Input: dimensioned drawing with shaded views. Units: mm. Origin: part minimum x, y, z. A direction names the side the tool comes from. Round coordinates to 2 decimals unless told otherwise and drop trailing zeros. Order: outer loops, then holes, each group sorted by start corner. A loop starts at its lowest first (then second) coordinate and runs counter-clockwise, first axis right, second up. Notation, with made-up numbers: M -6.75,-16.75 L 51.25,-16.75 A38 ccw 51.25,21.25 Z; hole C 89,27.25 d10. An arc over 180 degrees is marked long. Use one line per item in the form item = value. Start each with the question number.
Q1. Section D-D (z = 15). Return the cut outline in (x, y).
Q2. Reachability of the marked faces 1 and 2 from +Z, -Z, +X, -X, +Y, -Y: full face, straight path, thin tool, end or side. Return the list, or none.
Q3. Material intervals for probe 1 along Y at (x, z) = (29, 3.25); probe 2 along Z at (x, y) = (13, 50); probe 3 along X at (y, z) = (34, 16), sorted ascending.
Q4. Section C-C (z = 44). Return the cut outline in (x, y).
Q5. Section A-A (x = 29). Return the cut outline in (y, z).
Q6. Contact query for flat-ended pins moving along their axis: pin 1 (10 mm diameter, centred on x = 12.5, z = 22.5, fed in from +Y); pin 2 (1 mm diameter, centred on x = 50.5, y = 19, fed in from +Z); pin 3 (1 mm diameter, centred on y = 50, z = 25.5, fed in from -X). Output: stop coordinate, or through.
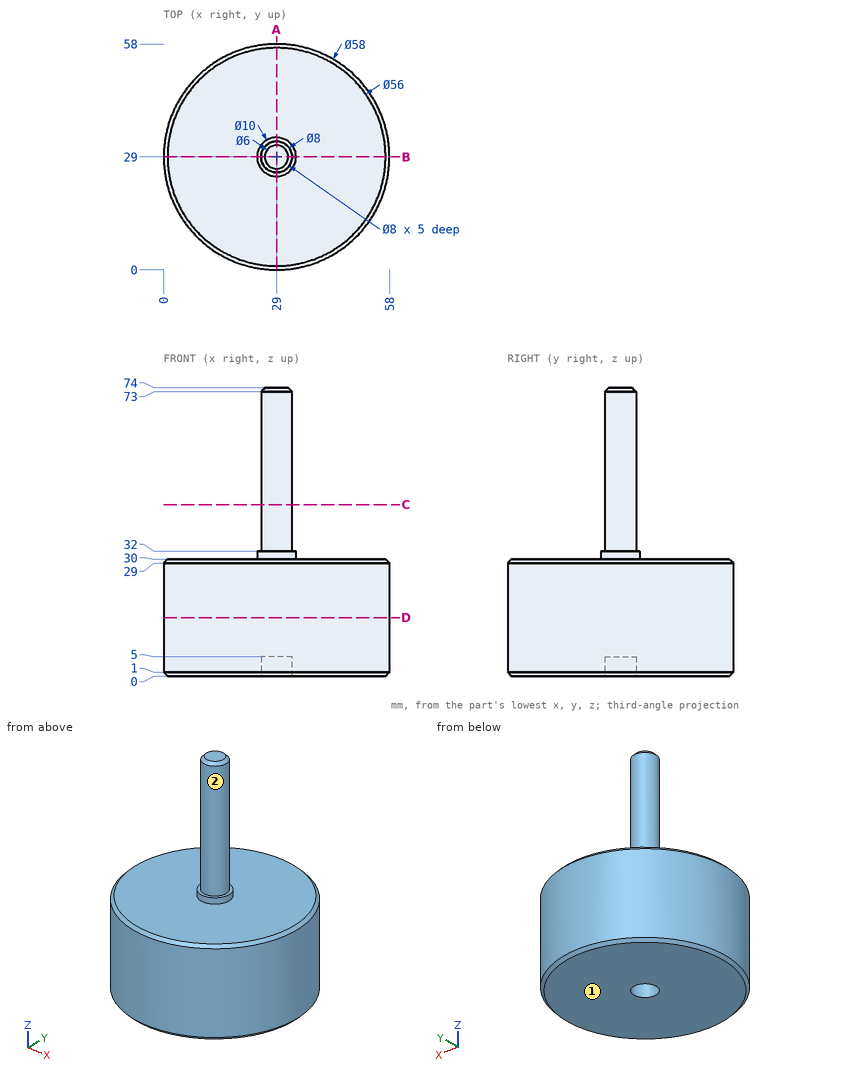
Results list:
q1.outline = C 29,29 d58
q2.face_1 = -Z, +X, -X, +Y, -Y
q2.face_2 = +Z
q3.probe_1 = 0 to 25, 33 to 58
q3.probe_2 = 0 to 30
q3.probe_3 = 0.43 to 57.57
q4.outline = C 29,29 d8
q5.outline = M 0,1 L 1,0 L 25,0 L 25,5 L 33,5 L 33,0 L 57,0 L 58,1 L 58,29 L 57,30 L 34,30 L 34,32 L 33,32 L 33,73 L 32,74 L 26,74 L 25,73 L 25,32 L 24,32 L 24,30 L 1,30 L 0,29 Z
q6.pin_1 = 55.62
q6.pin_2 = 30
q6.pin_3 = 8.49
